The listing builds one solid part. Answer for the finished solid, in the listing's coordinates (mm). A direction names the side the tool comes from. Round coordinates to 2 decimals unless told otherwise and drop trailing zeros. Write each loop counter-clockwise with the first axis right and the second up, starting at its lowest first coordinate (ties: lowest second). Pieces come first, ordered by that corner, then holes. Notation, with made-up numbers: M 63.5,11 L 107.5,11 A23 cw 107.5,46 Z; hole C -4.5,7.5 d1. An arc over 180 degrees is marked long. Answer as CSV lines item,"result". Start each with the question number.
from build123d import *

# Parameters (mm, degrees)
TABAN_FLAN_1_DEPTH    = 34
IZIM9_W               = 9.15
IZIM9_H               = 8
IZIM9_H_2             = 19
KES_EKSTR_ZYON1_DEPTH = 39.757096124
IZIM11_R              = 2.25
KES_EKSTR_ZYON2_DEPTH = 10
RADYUS1_SIZE          = 6


# Sheet-metal steps are written as plain solids
with BuildPart() as part:
    # Çizim1 → Taban-Flanş1 (new, symmetric)
    with BuildSketch(Plane.XY):
        with BuildLine():
            Line((-12.5, 0), (12.5, 0))
            ThreePointArc((12.5, 0), (14.537154879, -7.765591238), (8.95035213, -2))
            Line((8.95035213, -2), (10.233357384, -2.777108434))
            ThreePointArc((10.233357384, -2.777108434), (13.800833838, -6.458751031), (12.5, -1.5))
            Line((12.5, -1.5), (-12.5, -1.5))
            Line((-12.5, -1.5), (-12.5, 0))
        make_face()
    extrude(amount=TABAN_FLAN_1_DEPTH, both=True)

    # Çizim9 → Kes-Ekstrüzyon1 (cut, through all)
    with BuildSketch(Plane(origin=(0, 0, 0), x_dir=(1, 0, 0), z_dir=(0, 1, 0))):
        with Locations((12.075, 30)):
            Rectangle(IZIM9_W, IZIM9_H)
        with Locations((12.075, -30)):
            Rectangle(IZIM9_W, IZIM9_H)
        with Locations((12.075, 0)):
            Rectangle(IZIM9_W, IZIM9_H_2)
    extrude(amount=-KES_EKSTR_ZYON1_DEPTH, mode=Mode.SUBTRACT)

    # Çizim11 → Kes-Ekstrüzyon2 (cut)
    with BuildSketch(Plane(origin=(0, 0, 0), x_dir=(1, 0, 0), z_dir=(0, 1, 0))):
        with Locations(Location((-1, 25, 0), (0, 0, 180))):
            Circle(IZIM11_R)
        with Locations(Location((-1, -25, 0), (0, 0, 180))):
            Circle(IZIM11_R)
        with Locations(Location((-5, 0, 0), (0, 0, 180))):
            Circle(IZIM11_R)
    extrude(amount=-KES_EKSTR_ZYON2_DEPTH, mode=Mode.SUBTRACT)

    # Radyus1
    radyus1_edges = [part.edges().sort_by_distance(p)[0] for p in [
        (-12.5, -0.75, 34),
        (-12.5, -0.75, -34),
    ]]
    chamfer(radyus1_edges, length=RADYUS1_SIZE)


solid = part.part
Q1. Each of these flat-tipped pins is pushed along its axis until it touches: P1, Ø7, axis at x = -1, z = -25, coming from the -Y side; P2, Ø1.6, axis at y = -1, z = -31, coming from the +X side; P3, Ø2.5, axis at x = 10, y = -5, coming from the -Z side. Where does it stop, or does it pass through?
Q2. Find section B-B (z = -25). Determine the outline of the cut face in (x, y), plus the area to 3 significant figures.
Q3. Find section A-A (y = -4.15). Determine the outline of the cut face in (x, z).
Q4. The mould has two halves that part along Z. Classify faces 1 (the face through (-0.512, -0.74, -27.196)), 2 (the face through (0, -1.5, 0)), 3 (the face through (1, -1, 34)): +Z half, -Z half, draft (parallel to the pull), parting line (faces both ways), or undercut.
Q5. Find section D-D (x = -1). Determine the outline of the cut face in (y, z), plus the area to 3 significant figures.
Q6. For faces 4 (the face through (12, -1, 26)), 5 (the face through (7.5, -1, -30)), 6 (the face through (9.58, -2.38, -17.63)), determine the directions among +Z, -Z, +X, -X, +Y, -Y from which every point of the face is accessible in a straight line to the end or side of a thin tool.
Q7. Find section C-C (x = -5). Determine the outline of the cut face in (y, z), plus the area to 4 significant figures.
Q8. Straight lines are drawn through the part: L1, parallel to Z at x = -1, y = -0.4; L2, parallel to Y at x = 12.5, z = -22.5; L3, parallel to X at y = -4.15, z = -20.25. For each, find the intervals that lie inside material, in ascending order.
Reported:
1,P1,"stops at y = -1.5"
1,P2,"stops at x = 7.5"
1,P3,"stops at z = -26"
2,outline,"M -12.5,-1.5 L -3.25,-1.5 L -3.25,0 L -12.5,0 Z; M 1.25,-1.5 L 12.5,-1.5 A2.65 cw long 10.23,-2.78 L 8.95,-2 A4.15 ccw long 12.5,0 L 1.25,0 Z"
2,area,"57.6 mm2"
3,outline,"M 8.35,-26 L 9.85,-26 L 9.85,-9.5 L 8.35,-9.5 Z; M 8.35,9.5 L 9.85,9.5 L 9.85,26 L 8.35,26 Z; M 15.15,-26 L 16.65,-26 L 16.65,-9.5 L 15.15,-9.5 Z; M 15.15,9.5 L 16.65,9.5 L 16.65,26 L 15.15,26 Z"
4,face 1,"undercut"
4,face 2,"draft"
4,face 3,"+Z half"
5,outline,"M -1.5,-34 L 0,-34 L 0,-27.25 L -1.5,-27.25 Z; M -1.5,-22.75 L 0,-22.75 L 0,22.75 L -1.5,22.75 Z; M -1.5,27.25 L 0,27.25 L 0,34 L -1.5,34 Z"
5,area,"88.5 mm2"
6,face 4,"+Z, +X, +Y, -Y"
6,face 5,"-Z, +X, +Y, -Y"
6,face 6,"+Z, -Z"
7,outline,"M -1.5,-34 L 0,-34 L 0,-2.25 L -1.5,-2.25 Z; M -1.5,2.25 L 0,2.25 L 0,34 L -1.5,34 Z"
7,area,"95.25 mm2"
8,L1,"z = -34 to -27.25, -22.75 to 22.75, 27.25 to 34"
8,L2,"y = -8.3 to -6.8, -1.5 to 0"
8,L3,"x = 8.35 to 9.85, 15.15 to 16.65"
